Check sheet for the modelled part. Datum: model origin and axes. Units: mm. Face numbers are marked on the shaded views. A direction names the side the tool comes from. Coordinates: 2 decimals unless noted, no trailing zeros. Write each loop counter-clockwise with the first axis right and the second up, starting at its lowest first coordinate (ties: lowest second). Pieces come first, ordered by that corner, then holes. Notation, with made-up numbers: M 25,32 L 33,32 A10 ccw 33,45 Z; hole C 36.5,87.25 d4. An arc over 180 degrees is marked long. Answer as CSV lines item,"result".
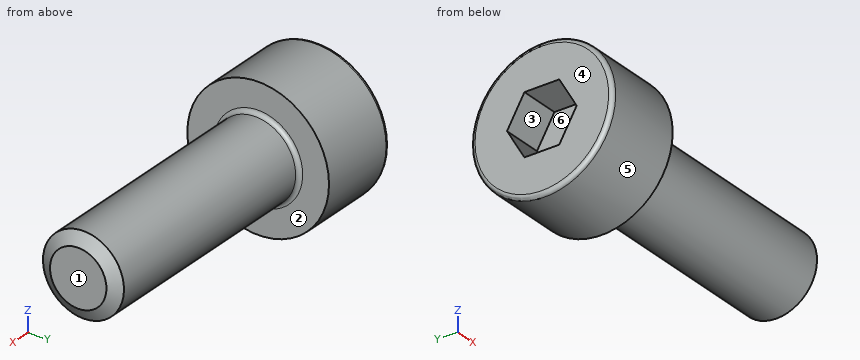
from build123d import *

# Parameters (mm, degrees)
SKETCH_1_W          = 4
SKETCH_1_H          = 3.5
SKETCH_2_R          = 2
EXTRUDE_1_DEPTH     = 12
CUT_EXTRUDE_1_DEPTH = 2
CHAMFER_1_SIZE      = 0.6062
CHAMFER_1_SIZE2     = 0.35
FILLET_1_R          = 0.2


with BuildPart() as part:
    # 草图1 → 旋转1 (revolve)
    with BuildSketch(Plane.XY):
        with Locations((2, 1.75)):
            Rectangle(SKETCH_1_W, SKETCH_1_H)
    revolve(axis=Axis((0, 0, 0), (1, 0, 0)))

    # 草图2 → 凸台-拉伸1 (add)
    with BuildSketch(Plane(origin=(4, 0, 0), x_dir=(0, 0, -1), z_dir=(1, 0, 0))):
        Circle(SKETCH_2_R)
    extrude(amount=EXTRUDE_1_DEPTH)

    # 草图3 → 切除-拉伸1 (cut)
    with BuildSketch(Plane.ZY):
        Polygon((0, 1.72), (-1.489563695, 0.86), (-1.489563695, -0.86), (0, -1.72), (1.489563695, -0.86), (1.489563695, 0.86), align=None)
    extrude(amount=-CUT_EXTRUDE_1_DEPTH, mode=Mode.SUBTRACT)

    # 倒角1
    chamfer_1_edges = [part.edges().sort_by_distance(p)[0] for p in [
        (16, 0, 2),
    ]]
    chamfer_1_side = [part.faces().sort_by_distance(p)[0] for p in [
        (16, 0, 0),
    ]]
    chamfer(chamfer_1_edges, length=CHAMFER_1_SIZE, length2=CHAMFER_1_SIZE2, reference=chamfer_1_side[0])

    # 圆角1
    fillet_1_edges = [part.edges().sort_by_distance(p)[0] for p in [
        (0, -3.5, 0),
        (4, 0, 2),
    ]]
    fillet(fillet_1_edges, radius=FILLET_1_R)


solid = part.part
1) Tool access check on the marked faces 1, 2 and 3. Record the directions out of +Z, -Z, +X, -X, +Y, -Y that give a thin tool (end or side, any length) a straight path to the whole face; none if there is none.
Answer key:
face 1,"+Z, -Z, +X, +Y, -Y"
face 2,"+X"
face 3,"-X"
2) Section check B-B, the plane x = 2.5. Record the boundary of the cut face in (y, z), plus the area to 3 significant figures.
Answer key:
outline,"C 0,0 d7"
area,"38.5 mm2"
3) Thickness scan on line 1 along Y through (x, z) = (11, 0); line 2 along X through (y, z) = (-2.75, 0); line 3 along Z through (x, y) = (12, 0.5). Record the ranges inside material, lowest first.
Answer key:
line 1,"y = -2 to 2"
line 2,"x = 0 to 4"
line 3,"z = -1.94 to 1.94"
4) Depth check by flat-ended pin: P1, Ø1, axis at y = -1, z = -2, coming from the +X side; P2, Ø1.5, axis at y = 0, z = -0.5, coming from the -X side; P3, Ø1.5, axis at x = 11, z = 1, coming from the -Y side. Enter the tip coordinate at first touch or a pass-through.
Answer key:
P1,"stops at x = 15.8"
P2,"stops at x = 2"
P3,"stops at y = -1.98"
5) Section check A-A, the plane y = 0. Record the boundary of the cut face in (x, z), plus the area to 3 significant figures.
Answer key:
outline,"M 0,-3.3 A0.2 ccw 0.2,-3.5 L 4,-3.5 L 4,-2.2 A0.2 cw 4.2,-2 L 15.65,-2 L 16,-1.39 L 16,1.39 L 15.65,2 L 4.2,2 A0.2 cw 4,2.2 L 4,3.5 L 0.2,3.5 A0.2 ccw 0,3.3 L 0,1.49 L 2,1.49 L 2,-1.49 L 0,-1.49 Z"
area,"69.8 mm2"
6) Section check C-C, the plane x = 4.75. Record the boundary of the cut face in (y, z), plus the area to 3 significant figures.
Answer key:
outline,"C 0,0 d4"
area,"12.6 mm2"
7) Mould release check, pull along Y, two halves, no side actions. Record for the marked faces 4, 5 and 6: pulls with the +Y half, pulls with the -Y half, needs draft (parallel to the pull), parting line crosses it, or undercut.
Answer key:
face 4,"needs draft"
face 5,"parting line crosses it"
face 6,"undercut"
